Input: part model. Units: mm. Frame: model coordinates. Face numbers are marked on the shaded views. Give positions to 0.01 mm unless a question says otherwise; leave off trailing zeros. Loops run counter-clockwise (first coordinate to the right, second up) from the corner with the lowest first, then second, coordinate; pieces in that order, holes last.
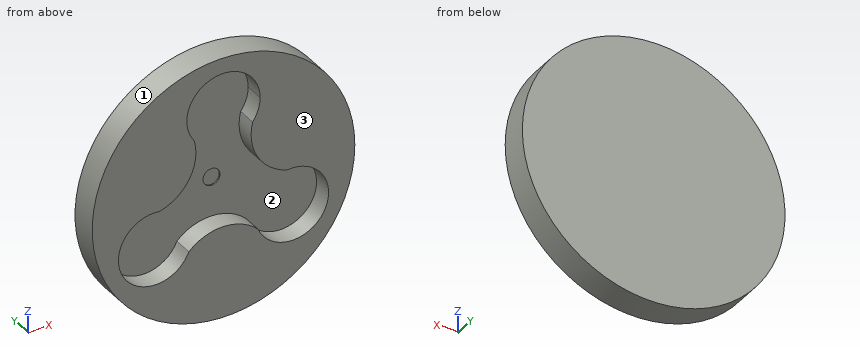
from build123d import *

# Parameters (mm, degrees)
F0_R     = 46.3668582169
F1_DEPTH = 10
F0_R_2   = 12.95
F0_R_3   = 10.95
F0_R_4   = 3
F2_DEPTH = 3
F0_R_5   = 2.5
F3_DEPTH = 2.5


with BuildPart() as f1:
    # F0 (on Front) → F1 (new body)
    with BuildSketch(Plane.XZ):
        Circle(F0_R)
        with BuildLine():
            ThreePointArc((-10.3030346023, 20.0546205966), (-4.1399397278, 40.1704278267), (12.95, 27.9))
            ThreePointArc((12.95, 27.9), (12.2704278267, 23.7600602722), (10.3030346023, 20.0546205966))
            ThreePointArc((10.3030346023, 20.0546205966), (12.0696833018, 6.9684349033), (22.5193282011, -1.1046205966))
            ThreePointArc((22.5193282011, -1.1046205966), (32.7186411149, -4.2294931122), (37.1121087656, -13.95))
            ThreePointArc((37.1121087656, -13.95), (26.7120297045, -26.6464720771), (12.2162935988, -18.95))
            ThreePointArc((12.2162935988, -18.95), (0, -13.9368698067), (-12.2162935988, -18.95))
            ThreePointArc((-12.2162935988, -18.95), (-35.3771377446, -20.425), (-22.5193282011, -1.1046205966))
            ThreePointArc((-22.5193282011, -1.1046205966), (-12.0696833018, 6.9684349033), (-10.3030346023, 20.0546205966))
        make_face(mode=Mode.SUBTRACT)
    extrude(amount=F1_DEPTH)

    # F0 (on Front) → F2 (join)
    with BuildSketch(Plane.XZ):
        with BuildLine():
            ThreePointArc((10.3030346023, 20.0546205966), (0, 14.95), (-10.3030346023, 20.0546205966))
            ThreePointArc((-10.3030346023, 20.0546205966), (-12.0696833018, 6.9684349033), (-22.5193282011, -1.1046205966))
            ThreePointArc((-22.5193282011, -1.1046205966), (-14.4416018778, -5.3934676507), (-11.2121087656, -13.95))
            ThreePointArc((-11.2121087656, -13.95), (-11.4656366885, -16.4999209389), (-12.2162935988, -18.95))
            ThreePointArc((-12.2162935988, -18.95), (0, -13.9368698067), (12.2162935988, -18.95))
            ThreePointArc((12.2162935988, -18.95), (12.9470797866, -7.475), (22.5193282011, -1.1046205966))
            ThreePointArc((22.5193282011, -1.1046205966), (12.0696833018, 6.9684349033), (10.3030346023, 20.0546205966))
        make_face()
        Circle(F0_R_2, mode=Mode.SUBTRACT)
        Circle(F0_R_2)
        Circle(F0_R_3, mode=Mode.SUBTRACT)
        with BuildLine():
            ThreePointArc((10.3030346023, 20.0546205966), (12.2704278267, 23.7600602722), (12.95, 27.9))
            ThreePointArc((12.95, 27.9), (-4.1399397278, 40.1704278267), (-10.3030346023, 20.0546205966))
            ThreePointArc((-10.3030346023, 20.0546205966), (0, 14.95), (10.3030346023, 20.0546205966))
        make_face()
        with Locations((0, 27.9)):
            Circle(F0_R_3, mode=Mode.SUBTRACT)
        with BuildLine():
            ThreePointArc((37.1121087656, -13.95), (32.7186411149, -4.2294931122), (22.5193282011, -1.1046205966))
            ThreePointArc((22.5193282011, -1.1046205966), (12.9470797866, -7.475), (12.2162935988, -18.95))
            ThreePointArc((12.2162935988, -18.95), (26.7120297045, -26.6464720771), (37.1121087656, -13.95))
        make_face()
        with Locations((24.1621087656, -13.95)):
            Circle(F0_R_3, mode=Mode.SUBTRACT)
        with BuildLine():
            ThreePointArc((-11.2121087656, -13.95), (-14.4416018778, -5.3934676507), (-22.5193282011, -1.1046205966))
            ThreePointArc((-22.5193282011, -1.1046205966), (-35.3771377446, -20.425), (-12.2162935988, -18.95))
            ThreePointArc((-12.2162935988, -18.95), (-11.4656366885, -16.4999209389), (-11.2121087656, -13.95))
        make_face()
        with Locations((-24.1621087656, -13.95)):
            Circle(F0_R_3, mode=Mode.SUBTRACT)
        Circle(F0_R_3)
        Circle(F0_R_4, mode=Mode.SUBTRACT)
        with Locations((0, 27.9)):
            Circle(F0_R_3)
        with Locations((24.1621087656, -13.95)):
            Circle(F0_R_3)
        with Locations((-24.1621087656, -13.95)):
            Circle(F0_R_3)
    extrude(amount=F2_DEPTH)

    # F0 (on Front) → F3 (join)
    with BuildSketch(Plane.XZ):
        Circle(F0_R)
        with BuildLine():
            ThreePointArc((-10.3030346023, 20.0546205966), (-4.1399397278, 40.1704278267), (12.95, 27.9))
            ThreePointArc((12.95, 27.9), (12.2704278267, 23.7600602722), (10.3030346023, 20.0546205966))
            ThreePointArc((10.3030346023, 20.0546205966), (12.0696833018, 6.9684349033), (22.5193282011, -1.1046205966))
            ThreePointArc((22.5193282011, -1.1046205966), (32.7186411149, -4.2294931122), (37.1121087656, -13.95))
            ThreePointArc((37.1121087656, -13.95), (26.7120297045, -26.6464720771), (12.2162935988, -18.95))
            ThreePointArc((12.2162935988, -18.95), (0, -13.9368698067), (-12.2162935988, -18.95))
            ThreePointArc((-12.2162935988, -18.95), (-35.3771377446, -20.425), (-22.5193282011, -1.1046205966))
            ThreePointArc((-22.5193282011, -1.1046205966), (-12.0696833018, 6.9684349033), (-10.3030346023, 20.0546205966))
        make_face(mode=Mode.SUBTRACT)
        Circle(F0_R_4)
        Circle(F0_R_5, mode=Mode.SUBTRACT)
        Circle(F0_R_5)
    extrude(amount=F3_DEPTH)


solid = f1.part
(1) Mould query, pull axis Z, two halves, no side actions, for the marked faces 1, 2 and 3. Classes: +Z half, -Z half, draft (parallel to the pull), parting line (faces both ways), or undercut.
Values follow:
face 1: parting line
face 2: undercut
face 3: draft
(2) Cut plane A-A (x = 0). Return the cut outline in (y, z), and give its area (3 significant figures).
Values follow:
outline: (-10, -46.37) - (0, -46.37) - (0, 46.37) - (-10, 46.37) - (-10, 40.85) - (-3, 40.85) - (-3, 3) - (-2.5, 3) - (-2.5, -3) - (-3, -3) - (-3, -13.94) - (-10, -13.94) - close
area: 541 mm2
(3) Ray query, probe 1 along X at (y, z) = (-8, -22); probe 2 along Z at (x, y) = (0, -2.9); probe 3 along X at (y, z) = (-8.25, -19.5). Return the intervals inside material, ascending.
Values follow:
probe 1: x = -40.82 to -34.31, -14.02 to 14.02, 34.31 to 40.82
probe 2: z = -46.37 to -3, 3 to 46.37
probe 3: x = -42.07 to -35.86, -12.46 to 12.46, 35.86 to 42.07
(4) Cut plane D-D (z = 12). Return the cut outline in (x, y), and give its area (3 significant figures).
Values follow:
outline: (-44.79, -10) - (-10.13, -10) - (-10.13, -3) - (10.13, -3) - (10.13, -10) - (44.79, -10) - (44.79, 0) - (-44.79, 0) - close
area: 754 mm2
(5) Pin query (flat end, axial travel): pin 1 Ø23.5 at (x, z) = (24.16, -13.95) entering from -Y; pin 2 Ø5 at (x, y) = (23, -5) entering from +Z; pin 3 Ø3 at (x, y) = (28.5, -3) entering from +Z. Return the tip coordinate at first contact, or that it passes through.
Values follow:
pin 1: stops at y = -3
pin 2: stops at z = 41.59
pin 3: stops at z = 37.69
(6) Cut plane B-B (z = 30.5). Return the cut outline in (x, y).
Values follow:
outline: (-34.92, -10) - (-12.69, -10) - (-12.69, -3) - (12.69, -3) - (12.69, -10) - (34.92, -10) - (34.92, 0) - (-34.92, 0) - close
(7) Cut plane C-C (y = -6.75). Return the cut outline in (x, z).
Values follow:
outline: circle Ø92.73 at (0, 0); hole (-22.52, -1.1) arc R12.95 ccw (long way) to (-12.22, -18.95) arc R17.39 cw to (12.22, -18.95) arc R12.95 ccw (long way) to (22.52, -1.1) arc R17.39 cw to (10.3, 20.05) arc R12.95 ccw (long way) to (-10.3, 20.05) arc R17.39 cw to start
